Autodesk Inventor part; units mm, degrees
ref_plane "YZ Plane" through (0, 0, 0) normal (1, 0, 0) x (0, 1, 0)
ref_plane "XZ Plane" through (0, 0, 0) normal (0, 1, 0) x (-1, 0, 0)
ref_plane "XY Plane" through (0, 0, 0) normal (0, 0, 1) x (1, 0, 0)
sketch "Sketch1" plane through (0, 0, 0) normal (0, 1, 0) x (-1, 0, 0)
  point P0 (0, 0)
sketch "Sketch2" plane through (0, 0, 0) normal (0, 1, 0) x (-1, 0, 0)
  line L0 (0, 0) -> (25.4, 0)
  line L1 (25.4, 0) -> (25.4, -25.4)
  line L2 (25.4, -25.4) -> (0, -25.4)
  line L3 (0, -25.4) -> (0, 0)
  dimension "d0" = 25.4
  dimension "d1" = 25.4
extrude "Extrusion1" add sketch "Sketch2" along normal blind 17.78
sketch "Sketch3" plane through (0, 17.78, 0) normal (0, 1, 0) x (1, 0, 0)
  line L0 (-22.225, 3.175) -> (-3.175, 3.175)
  line L1 (-3.175, 3.175) -> (-3.175, 22.225)
  line L2 (-3.175, 22.225) -> (-22.225, 22.225)
  line L3 (-22.225, 22.225) -> (-22.225, 3.175)
  line L4 (-25.4, 25.4) -> (-25.4, 0)
  line L5 (0, 25.4) -> (-25.4, 25.4)
  line L6 (-25.4, 0) -> (0, 0)
  line L7 (0, 0) -> (0, 25.4)
  dimension "d4" = 3.175
  dimension "d5" = 3.175
  dimension "d6" = 3.175
  dimension "d7" = 3.175
extrude "Extrusion2" cut sketch "Sketch3" against normal blind 15.24 contours L3 L2 L1 L0
sketch "Sketch4" plane through (-25.4, 0, 0) normal (0, 0, 1) x (1, 0, 0)
  circle A0 centre (1.905, 16.51) radius 1.27
  circle A1 centre (23.495, 16.51) radius 1.27
  line L0 (0, 17.78) -> (25.4, 17.78)
  line L1 (3.175, 17.78) -> (3.175, 2.54)
  line L2 (22.225, 17.78) -> (22.225, 2.54)
  line L3 (3.175, 17.78) -> (1.905, 17.78)
  line L4 (1.905, 17.78) -> (1.905, 12.446)
  line L5 (1.905, 12.446) -> (3.175, 12.446)
  line L6 (3.175, 12.446) -> (3.175, 17.78)
  line L7 (22.225, 17.78) -> (23.495, 17.78)
  line L8 (23.495, 17.78) -> (23.495, 12.446)
  line L9 (23.495, 12.446) -> (22.225, 12.446)
  line L10 (22.225, 12.446) -> (22.225, 17.78)
  line L11 (3.175, 17.78) -> (0, 17.78)
  line L12 (0, 17.78) -> (0, 12.446)
  line L13 (0, 12.446) -> (3.175, 12.446)
  line L14 (3.175, 12.446) -> (3.175, 17.78)
  line L15 (22.225, 17.78) -> (25.4, 17.78)
  line L16 (25.4, 17.78) -> (25.4, 12.446)
  line L17 (25.4, 12.446) -> (22.225, 12.446)
  line L18 (22.225, 12.446) -> (22.225, 17.78)
  point P0 (25.4, 0)
  point P1 (1.905, 12.446)
  point P2 (1.905, 15.24)
  point P3 (1.905, 17.78)
  point P4 (23.495, 15.24)
  dimension "d10" = 2.54
  dimension "d11" = 2.54
  dimension "d12" = 1.27
  dimension "d13" = 1.27
  dimension "d14" = 1.27
  dimension "d15" = 1.27
  dimension "d16" = 1.27
  dimension "d17" = 5.334
  dimension "d18" = 1.27
  dimension "d19" = 5.334
extrude "Extrusion3" cut sketch "Sketch4" against normal blind 25.4 contours A0 L4 L13 L12 L0 | L0 L16 L17 L8 A1
sketch "Sketch5" plane through (0, 0, 0) normal (1, 0, 0) x (0, 0, -1)
  line L0 (3.175, 17.78) -> (22.225, 17.78)
  line L1 (0, 12.446) -> (25.4, 12.446)
  line L2 (0, 12.446) -> (25.4, 12.446)
  line L3 (0, 17.78) -> (3.675, 17.78)
  line L4 (3.675, 17.78) -> (3.675, 12.446)
  line L5 (3.675, 12.446) -> (0, 12.446)
  line L6 (0, 12.446) -> (0, 17.78)
  line L7 (25.4, 15.24) -> (25.4, 17.78)
  line L8 (25.4, 17.78) -> (21.725, 17.78)
  line L9 (21.725, 17.78) -> (21.725, 12.446)
  line L10 (21.725, 12.446) -> (25.4, 12.446)
  line L11 (25.4, 12.446) -> (25.4, 17.78)
  line L12 (22.225, 2.54) -> (3.175, 2.54)
  line L13 (3.675, 12.446) -> (3.175, 12.446)
  line L14 (3.175, 12.446) -> (3.175, 2.54)
  line L15 (3.175, 2.54) -> (3.675, 2.54)
  line L16 (3.675, 2.54) -> (3.675, 12.446)
  line L17 (22.225, 17.78) -> (22.225, 2.54)
  line L18 (21.725, 12.446) -> (22.225, 12.446)
  line L19 (22.225, 12.446) -> (22.225, 2.54)
  line L20 (22.225, 2.54) -> (21.725, 2.54)
  line L21 (21.725, 2.54) -> (21.725, 12.446)
  point P0 (0, 0)
  point P1 (25.4, 12.446)
  point P2 (21.725, 12.446)
  point P3 (0, 12.446)
  point P4 (22.225, 12.446)
  dimension "d25" = 3.675
  dimension "d26" = 3.675
extrude "Extrusion4" cut sketch "Sketch5" against normal blind 25.4 contours L0 L4 L1 L6 L3 | L0 L17 L1 L9 | L16 L12 L14 L1 | L8 L7 L11 L1 L17 | L1 L17 L12 L21
sketch "Sketch7" plane through (0, 2.54, -3.675) normal (0, 0, 1) x (1, 0, 0)
  line L0 (-3.175, 15.24) -> (-3.175, 0)
  line L1 (-1.905, 12.7) -> (-1.905, 9.906)
  line L2 (0, 9.906) -> (0, 0)
  line L3 (-1.905, 9.906) -> (0, 9.906)
  line L4 (0, 0) -> (-1.905, 9.906)
  line L5 (-1.905, 9.906) -> (0, 9.906)
  line L6 (0, 0) -> (-25.4, 0)
  line L7 (0, 0) -> (0, 9.906)
  line L8 (0, 9.906) -> (-25.4, 9.906)
  line L9 (-25.4, 9.906) -> (-25.4, 0)
  line L10 (-23.495, 9.906) -> (-23.495, 12.7)
  line L11 (-25.4, 0) -> (-23.495, 9.906)
  line L12 (-23.495, 9.906) -> (-25.4, 9.906)
  point P0 (0, -2.54)
extrude "Extrusion6" cut sketch "Sketch7" against normal blind 18.5 contours L3 L2 L4 | L11 L9 L8
sketch "Sketch8" plane through (-23.495, 17.78, -3.675) normal (0, 0, 1) x (1, 0, 0)
  arc A0 (0, 0) -> (0, -2.54) centre (0, -1.27) ccw
  line L0 (-1.07, -2.27) -> (-1.07, 0)
  line L1 (-1.07, 0) -> (-1.27, 0)
  line L2 (-1.27, 0) -> (-1.27, -1.27)
  line L3 (-1.07, 0) -> (-1.07, -2.27)
  line L4 (-1.07, -2.27) -> (-1.27, -2.27)
  line L5 (-1.27, -2.27) -> (-1.27, -1.27)
  arc A1 (21.59, -2.54) -> (21.59, 0) centre (21.59, -1.27) ccw
  line L6 (22.66, -1.3632) -> (22.66, 0)
  line L7 (22.66, 0) -> (22.86, 0)
  line L8 (22.86, 0) -> (22.86, -1.27)
  line L9 (22.86, -1.3632) -> (22.86, -3.2076)
  line L10 (22.86, -3.2076) -> (22.66, -3.2076)
  line L11 (22.66, -3.2076) -> (22.66, -1.3632)
  line L12 (22.86, 0) -> (-1.27, 0)
  line L13 (-1.27, 0) -> (-1.27, -0.3)
  line L14 (-1.27, -0.3) -> (22.86, -0.3)
  line L15 (22.86, -0.3) -> (22.86, 0)
  line L16 (0, 0) -> (1.27, 0)
  point P0 (23.495, -17.78)
  point P1 (10.795, -0.3)
  point P2 (22.66, -1.9541)
  point P3 (22.66, -0.5859)
  point P4 (-1.07, 0)
  point P5 (-1.07, -0.3)
  point P6 (22.86, -0.3)
  point P7 (22.66, 0)
  dimension "d34" = 0.2
  dimension "d35" = 1
  dimension "d36" = 0.2
  dimension "d37" = 0.3
  dimension "d38" = 0
extrude "Extrusion7" cut sketch "Sketch8" against normal blind 18.5 contours L12 A1 L14 A0 | A0 L14 L0 L12 | L0 L14 L2 L1 | L0 A0 | A0 L2 L14 L0 | A1 L12 L6 L14 | A0 L0 L4 L5 | A1 L11 L6 | L6 L7 L8 L14
properties part number "boxtest2"
Work out the finished part from the listing and answer in its coordinate system (mm). A direction names the side the tool comes from. Give positions to 0.01 mm unless a question says otherwise; leave off trailing zeros. Loops run counter-clockwise (first coordinate to the right, second up) from the corner with the lowest first, then second, coordinate; pieces in that order, holes last. Notation, with made-up numbers: (4, -40) -> (19, -40) arc R11 ccw to (19, -36) -> close; hole circle Ø6 at (-4, 83.5). An arc over 180 degrees is marked (long way). Put each result on its own line as item: value. Start each with the question number.
Item 1: Each of these flat-tipped pins is pushed along its axis until it touches: P1, Ø0.8, axis at y = 13.5, z = -13, coming from the +X side (3 decimals); P2, Ø1.5, axis at x = -5.5, y = 14, coming from the +Z side; P3, Ø2, axis at y = 14, z = -17, coming from the -X side (3 decimals); P4, Ø2.5, axis at x = -7, z = -23.5, coming from the +Y side. Where does it stop, or does it pass through?
Item 2: The part is cut by section B-B (z = -19.5). Give the vertices of the cut face in (x, y) (3 decimals).
Item 3: The part is cut by section C-C (x = -10.25). Give the vertices of the cut face in (y, z) (3 decimals).
Item 4: The part is cut by section A-A (y = 13). Give the vertices of the cut face in (x, z) (3 decimals).
Item 5: The mould has two halves that part along X. Classify faces 1 (the face through (-25.4, 2, -13)), 2 (the face through (-3.175, 10, -13)), 3 (the face through (-13, 12.446, -2)): released by +X, released by -X, zero draft, split by the parting line, or undercut.
Item 6: Which of the six approach directions +Z, -Z, +X, -X, +Y, -Y give full straight-line access (tool end or side, diameter ignored) to faces 4 (the face through (-0.835, 17, -13)), 5 (the face through (-0.94, 7.42, -12.57)), 6 (the face through (-2, 10, -21.725)), 7 (the face through (-24.565, 17, -13)), 8 (the face through (-24.46, 7.42, -12.57))?
Item 7: The part is cut by section D-D (y = 5.25). Give the vertices of the cut face in (x, z) (3 decimals), then the cut area to 3 significant figures.
Item 8: Find the intervals of material crossed by L1, parallel to Z at x = -2, y = 10.5 (3 decimals); L2, parallel to X at y = 12.5, z = -7.25 (3 decimals); L3, parallel to Z at x = -15.75, y = 6.75 (3 decimals), in increasing order. Write a range as [from, to].
Answers below:
1. P1: x = -1.905
1. P2: through
1. P3: x = -23.495
1. P4: y = 12.45
2. outline: (-25.4, 0) -> (0, 0) -> (0, 2.54) -> (-1.905, 12.446) -> (-1.905, 15.24) arc R1.27 ccw to (-0.835, 15.826) -> (-0.835, 17.194) arc R1.27 ccw to (-1.085, 17.48) -> (-3.175, 17.48) -> (-3.175, 2.54) -> (-22.225, 2.54) -> (-22.225, 17.48) -> (-24.315, 17.48) arc R1.27 ccw to (-24.565, 17.194) -> (-24.565, 15.826) arc R1.27 ccw to (-23.495, 15.24) -> (-23.495, 12.446) -> (-25.4, 2.54) -> close
3. outline: (0, -25.4) -> (12.446, -25.4) -> (12.446, -22.225) -> (2.54, -22.225) -> (2.54, -3.175) -> (12.446, -3.175) -> (12.446, 0) -> (0, 0) -> close
4. outline: (-23.495, -21.725) -> (-22.225, -21.725) -> (-22.225, -3.675) -> (-23.495, -3.675) -> close; (-3.175, -21.725) -> (-1.905, -21.725) -> (-1.905, -3.675) -> (-3.175, -3.675) -> close
5. face 1: released by -X
5. face 2: undercut
5. face 3: zero draft
6. face 4: +Z, -Z, +X, +Y
6. face 5: +X
6. face 6: +X, -X, +Y
6. face 7: +Z, -Z, -X, +Y
6. face 8: -X
7. outline: (-25.4, -25.4) -> (0, -25.4) -> (0, -22.225) -> (-25.4, -22.225) -> close; (-25.4, -3.175) -> (0, -3.175) -> (0, 0) -> (-25.4, 0) -> close; (-24.879, -21.725) -> (-22.225, -21.725) -> (-22.225, -3.675) -> (-24.879, -3.675) -> close; (-3.175, -21.725) -> (-0.521, -21.725) -> (-0.521, -3.675) -> (-3.175, -3.675) -> close
7. area: 257 mm2
8. L1: [-25.4, -22.225], [-21.725, -3.675], [-3.175, 0]
8. L2: [-23.495, -22.225], [-3.175, -1.905]
8. L3: [-25.4, -22.225], [-3.175, 0]
